Geometry: final body of the model. Coordinates: model frame, mm. Give positions to 0.01 mm unless a question says otherwise; leave off trailing zeros. Order: outer loops, then holes, each group sorted by start corner. A loop starts at its lowest first (then second) coordinate and runs counter-clockwise, first axis right, second up. Notation, with made-up numbers: (-9.75, -27) -> (26.25, -27) arc R27 ccw to (26.25, -8) -> close; hole circle Ø3 at (43, -21.5). An arc over 180 degrees is marked (long way). Answer in a Markdown table with one row per item. Add a question column.
Q1. Cut plane A-A on x = 0. Return the cut outline in (y, z).
Q2. Pull-direction query (X, two-part tool) for faces 1 (the face through (0.715, -1.375, 0.177)), 2 (the face through (-6.5, 0, 1)), 3 (the face through (-2.579, -1.978, 1.187)), 4 (the face through (0, -6.5, 1)); classes: +X half, -X half, draft (parallel to the pull), parting line (faces both ways), or undercut.
Q3. Cut plane D-D on x = -2.5. Return the cut outline in (y, z), and give its area (3 significant figures).
Q4. Line query: line 1 along Y through (x, z) = (0, 1.25); line 2 along Y through (x, z) = (0, 0.2); line 3 along Z through (x, y) = (1.25, -1.5). Output: solid intervals per line, ascending. Write a range as from..to.
Q5. Contact query for a flat-ended pin moving along its axis: P1, Ø3, axis at x = 0.5, y = -1.5, coming from the +Z side. Output: stop coordinate, or through.
Q6. Cut plane C-C on z = 0.65. Return the cut outline in (x, y), and give its area (3 significant figures).
from build123d import *

# Parameters (mm, degrees)
F0_W     = 13
F0_H     = 13
F1_DEPTH = 2
F2_R     = 3.25
F3_DEPTH = 1.65
F4_R     = 1.55
F5_DEPTH = 1


with BuildPart() as f1:
    # F0 (on Top) → F1 (new body)
    with BuildSketch(Plane.XY):
        Rectangle(F0_W, F0_H)
    extrude(amount=F1_DEPTH)

    # F2 (on face) → F3 (cut)
    with BuildSketch(Plane.XY.offset(2)):
        Circle(F2_R)
    extrude(amount=-F3_DEPTH, mode=Mode.SUBTRACT)

    # F4 (on face) → F5 (cut)
    with BuildSketch(Plane.XY.offset(0.35)):
        Circle(F4_R)
    extrude(amount=-F5_DEPTH, mode=Mode.SUBTRACT)


solid = f1.part
Completed:
| question | item | result |
|---|---|---|
| 1 | outline | (-6.5, 0) -> (-1.55, 0) -> (-1.55, 0.35) -> (-3.25, 0.35) -> (-3.25, 2) -> (-6.5, 2) -> close; (1.55, 0) -> (6.5, 0) -> (6.5, 2) -> (3.25, 2) -> (3.25, 0.35) -> (1.55, 0.35) -> close |
| 2 | face 1 | undercut |
| 2 | face 2 | -X half |
| 2 | face 3 | undercut |
| 2 | face 4 | draft |
| 3 | outline | (-6.5, 0) -> (6.5, 0) -> (6.5, 2) -> (2.08, 2) -> (2.08, 0.35) -> (-2.08, 0.35) -> (-2.08, 2) -> (-6.5, 2) -> close |
| 3 | area | 19.1 mm² |
| 4 | line 1 | y = -6.5..-3.25, 3.25..6.5 |
| 4 | line 2 | y = -6.5..-1.55, 1.55..6.5 |
| 4 | line 3 | z = 0..0.35 |
| 5 | P1 | stops at z = 0.35 |
| 6 | outline | (-6.5, -6.5) -> (6.5, -6.5) -> (6.5, 6.5) -> (-6.5, 6.5) -> close; hole circle Ø6.5 at (0, 0) |
| 6 | area | 136 mm² |
